from build123d import *

# Parameters (mm, degrees)
SKETCH_1_R          = 1.5
SKETCH_1_R_2        = 2.9
SKETCH_1_R_3        = 13
EXTRUDE_2_DEPTH     = 2
EXTRUDE_3_DEPTH     = 3
SKETCH_3_R          = 9.847727686
SKETCH_3_R_2        = 8.997097943
SKETCH_3_R_3        = 10.721268195
SKETCH_3_R_4        = 10.991913459
SKETCH_3_R_5        = 8.225176043
SKETCH_3_R_6        = 6.770172336
CUT_EXTRUDE_1_DEPTH = 3


with BuildPart() as part:
    # 草图1 → 凸台-拉伸2 (new body)
    with BuildSketch(Plane.XY):
        with BuildLine():
            Line((49.779367134, 18.85), (49.779367134, 38.85))
            Line((49.779367134, 38.85), (-23.899828069, 88.85))
            Line((-23.899828069, 88.85), (-66.5, 88.85))
            Line((-66.5, 88.85), (-66.5, 28.68453606))
            Line((-66.5, 28.68453606), (-60.610760184, 25.264800383))
            Line((-60.610760184, 25.264800383), (-49.5, 18.85))
            ThreePointArc((-49.5, 18.85), (-61.52081528, 13.87081528), (-66.5, 1.85))
            Line((-66.5, 1.85), (-66.5, -7))
            Line((-66.5, -7), (-49.450486279, -7))
            Line((-49.450486279, -7), (-49.450486279, -16.236884808))
            Line((-49.450486279, -16.236884808), (49.779367134, -16.236884808))
            Line((49.779367134, -16.236884808), (49.779367134, -7))
            Line((49.779367134, -7), (66.779367134, -7))
            Line((66.779367134, -7), (66.779367134, 1.85))
            ThreePointArc((66.779367134, 1.85), (61.800182415, 13.87081528), (49.779367134, 18.85))
        make_face()
        with Locations((-61.3, 1.85)):
            Circle(SKETCH_1_R, mode=Mode.SUBTRACT)
        with Locations((-43.5, 13)):
            Circle(SKETCH_1_R, mode=Mode.SUBTRACT)
        with Locations((15, -8.15)):
            Circle(SKETCH_1_R_2, mode=Mode.SUBTRACT)
        with Locations((37.5, 30.82114317)):
            Circle(SKETCH_1_R_2, mode=Mode.SUBTRACT)
        with Locations((-60.344210129, 35.35)):
            Circle(SKETCH_1_R_2, mode=Mode.SUBTRACT)
        with Locations((-37.844210129, 74.32114317)):
            Circle(SKETCH_1_R_2, mode=Mode.SUBTRACT)
        with Locations((43.5, 13)):
            Circle(SKETCH_1_R, mode=Mode.SUBTRACT)
        with Locations((61.3, 1.85)):
            Circle(SKETCH_1_R, mode=Mode.SUBTRACT)
        with Locations((-49.094210129, 54.835571585)):
            Circle(SKETCH_1_R_3, mode=Mode.SUBTRACT)
    extrude(amount=EXTRUDE_2_DEPTH)

    # 草图2 → 凸台-拉伸3 (add)
    with BuildSketch(Plane.XY.offset(2)):
        Polygon((-1.860316433, 22.713601471), (-36.501332584, 42.713601471), (-32.501332584, 42.713601471), (2.139683567, 22.713601471), (20.139683567, 22.713601471), (20.139683567, 18.713601471), (2.139683567, 18.713601471), (-1.860316433, 18.713601471), (-19.860316433, 18.713601471), (-19.860316433, 22.713601471), align=None)
    extrude(amount=EXTRUDE_3_DEPTH)

    # 草图3 → 切除-拉伸1 (cut, through all)
    with BuildSketch(Plane.XY.offset(2)):
        with Locations((-23.384871699, 58.634182407)):
            Circle(SKETCH_3_R)
        with Locations((-3.787476222, 54.505622136)):
            Circle(SKETCH_3_R_2)
        with Locations((-29.351202297, 4.727480211)):
            Circle(SKETCH_3_R_3)
        with Locations((-2.325708947, 4.727480211)):
            Circle(SKETCH_3_R_4)
        with Locations((26.76200458, 6.974994395)):
            Circle(SKETCH_3_R_5)
        with Locations((17.040896101, 36.475624713)):
            Circle(SKETCH_3_R_6)
    extrude(amount=-CUT_EXTRUDE_1_DEPTH, mode=Mode.SUBTRACT)


solid = part.part
The model under review builds one solid part; all positions refer to its coordinate system, in mm. A direction names the side the tool comes from. Round coordinates to 2 decimals unless told otherwise and drop trailing zeros. Order: outer loops, then holes, each group sorted by start corner. A loop starts at its lowest first (then second) coordinate and runs counter-clockwise, first axis right, second up. Notation, with made-up numbers: (61, 22.25) - (68, 22.25) arc R13 cw to (68, 41.25) - close; hole circle Ø11 at (57, 26). An arc over 180 degrees is marked (long way). Use one line per item in the form item = value.
Q1. Add section C-C on x = 15. Give the boundary of the cut face in (y, z), then the cut area to 3 significant figures.
Response values:
outline = (-16.24, 0) - (-11.05, 0) - (-11.05, 2) - (-16.24, 2) - close; (-5.25, 0) - (30.02, 0) - (30.02, 2) - (22.71, 2) - (22.71, 5) - (18.71, 5) - (18.71, 2) - (-5.25, 2) - close; (42.93, 0) - (62.45, 0) - (62.45, 2) - (42.93, 2) - close
area = 132 mm^2
Q2. Tool access review of faces 4 (the flat face through (-63.6, 27, 1)), 5 (the flat face through (-18.938, 32.574, 3.479)), 6 (the cylindrical face through (-38.2, 77.2, 1)), 7 (the flat face through (-35, 42.714, 3)), 8 (the flat face through (-15.42, 32.85, 3.48)): name each direction out of +Z, -Z, +X, -X, +Y, -Y from which nothing blocks a thin tool from reaching the whole face with its end or side.
Response values:
face_4 = +Z, -Z, -X
face_5 = +Z, -X
face_6 = +Z, -Z
face_7 = +Z, +X, -X, +Y
face_8 = +Z, +X, +Y
Q3. Add section D-D on x = -22. Give the boundary of the cut face in (y, z).
Response values:
outline = (-16.24, 0) - (-3.08, 0) - (-3.08, 2) - (-16.24, 2) - close; (12.53, 0) - (48.88, 0) - (48.88, 2) - (36.65, 2) - (36.65, 5) - (34.34, 5) - (34.34, 2) - (12.53, 2) - close; (68.38, 0) - (87.56, 0) - (87.56, 2) - (68.38, 2) - close
Q4. Mouldability with a two-part tool opening along Y and no side actions: class faces 1 (the cylindrical face through (12.103, -8.022, 0.986)), 2 (the flat face through (20.14, 21, 3)), 3 (the flat face through (11, 22.714, 3)) as pulls with the +Y half, pulls with the -Y half, needs draft (parallel to the pull), parting line crosses it, or undercut.
Response values:
face_1 = undercut
face_2 = needs draft
face_3 = pulls with the +Y half
Q5. Clearance check with flat-ended pins moving along their axes: P1, Ø1.5, axis at x = 10.5, z = 4, coming from the +Y side; P2, Ø1, axis at y = 28.5, z = 1.5, coming from the +X side; P3, Ø1.5, axis at x = -34.5, z = 4, coming from the +Y side; P4, Ø2.5, axis at x = 61.3, y = 1.85, coming from the -Z side. State where each tip first meets the part, or that it passes through.
Response values:
P1 = 22.71
P2 = 49.78
P3 = 42.71
P4 = through
Q6. Add section B-B on x = -43.5. Give the boundary of the cut face in (y, z).
Response values:
outline = (-16.24, 0) - (11.5, 0) - (11.5, 2) - (-16.24, 2) - close; (14.5, 0) - (43.1, 0) - (43.1, 2) - (14.5, 2) - close; (66.57, 0) - (88.85, 0) - (88.85, 2) - (66.57, 2) - close
Q7. To check wall thickness, follow line 1 (X direction, y = 5, z = 0.2); line 2 (X direction, y = 35.5, z = 1.15); line 3 (Y direction, x = -11, z = 1.7). State the ranges of each line that lie inside material, in increasing order.
Response values:
line_1 = -66.21 to -40.07, -18.63 to -13.31, 8.66 to 18.78, 34.75 to 66.48
line_2 = -66.5 to -63.24, -57.45 to 10.34, 23.74 to 49.78
line_3 = -16.24 to -2.02, 11.48 to 49.13, 59.88 to 80.1
Q8. Add section A-A on z = 3.15. Give the boundary of the cut face in (x, y), then the cut area to 3 significant figures.
Response values:
outline = (-36.5, 42.71) - (-1.86, 22.71) - (-19.86, 22.71) - (-19.86, 18.71) - (20.14, 18.71) - (20.14, 22.71) - (2.14, 22.71) - (-32.5, 42.71) - close
area = 240 mm^2
